```python
from build123d import *

# Parameters (mm, degrees)
BOSS_EXTRUDE1_DEPTH = 3.5
FILLET2_R           = 5
SHELL1_START        = 1
SHELL1_DEPTH        = 1.5
CUT_EXTRUDE1_START  = -3.5
SKETCH2_R           = 1
CUT_EXTRUDE1_DEPTH  = 3.5


# Read off the part's stored shape, not the designer's step: Shell1
with BuildPart() as part:
    # Sketch1 → Boss-Extrude1 (new body)
    with BuildSketch(Plane.XY):
        Polygon((0, 0), (-47, 0), (-47, 15), (-45, 15), (-45, 5.5), (0, 5.5), align=None)
    extrude(amount=BOSS_EXTRUDE1_DEPTH)

    # Fillet2
    fillet2_edges = [part.edges().sort_by_distance(p)[0] for p in [
        (-47, 0, 1.75),
        (-45, 5.5, 1.75),
    ]]
    fillet(fillet2_edges, radius=FILLET2_R)

    # Shell1 outline → Shell1 (cut)
    with BuildSketch(Plane.XY.offset(SHELL1_START)):
        with BuildLine():
            Line((0, 4.5), (-40, 4.5))
            ThreePointArc((-40, 4.5), (-44.242640687, 6.257359313), (-46, 10.5))
            Line((-46, 10.5), (-46, 5))
            ThreePointArc((-46, 5), (-44.828427125, 2.171572875), (-42, 1))
            Line((-42, 1), (0, 1))
            Line((0, 1), (0, 4.5))
        make_face()
    extrude(amount=SHELL1_DEPTH, mode=Mode.SUBTRACT)

    # Sketch2 → Cut-Extrude1 (cut)
    with BuildSketch(Plane.XY.offset(3.5).offset(CUT_EXTRUDE1_START)):
        with Locations(Location((-3, 2.75, 0), (0, 0, 180))):
            Circle(SKETCH2_R)
        with Locations(Location((-5.375, 2.75, 0), (0, 0, 180))):
            Circle(SKETCH2_R)
        with Locations(Location((-7.75, 2.75, 0), (0, 0, 180))):
            Circle(SKETCH2_R)
    extrude(amount=CUT_EXTRUDE1_DEPTH, mode=Mode.SUBTRACT)


solid = part.part
```
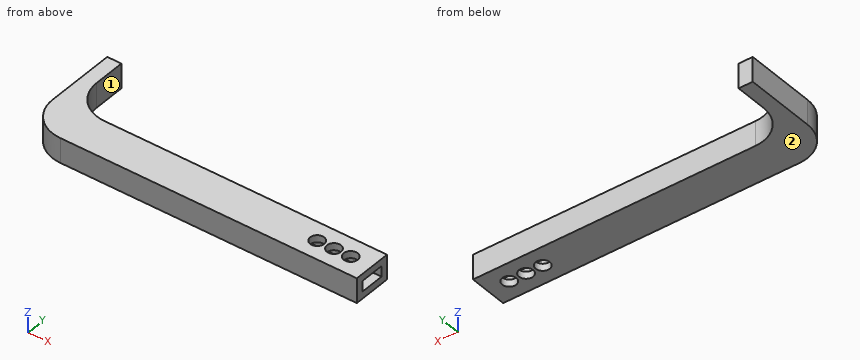
Work out the finished part from the listing and answer in its coordinate system (mm). Face numbers are marked on the shaded views. A direction names the side the tool comes from. Coordinates: 2 decimals unless noted, no trailing zeros. Write each loop counter-clockwise with the first axis right and the second up, starting at its lowest first coordinate (ties: lowest second). Pieces come first, ordered by that corner, then holes.
Q1. A cutting plane is placed at C-C, the plane z = 1.8. Give the vertices of the cut face in (x, y), then the cut area to 3 significant figures.
Q2. A cutting plane is placed at A-A, the plane x = -34.5. Give the vertices of the cut face in (y, z).
Q3. A cutting plane is placed at B-B, the plane y = 3.25. State how many separate pieces and enclosed holes the cut face has, then the cut area to 3 significant figures.
Q4. Which of the six approach directions +Z, -Z, +X, -X, +Y, -Y give full straight-line access (tool end or side, diameter ignored) to the marked faces 1 and 2?
Q5. Each of these flat-tipped pins is pushed along its axis until it touches: pin 1 Ø2.5 at (x, y) = (-3, 2.75) entering from -Z; pin 2 Ø1.8 at (x, z) = (-26.5, 2) entering from +Y; pin 3 Ø1.8 at (x, y) = (-5.375, 2.75) entering from +Z; pin 4 Ø1.2 at (y, z) = (7.5, 1.5) entering from +X. Where does it stop, or does it pass through?
Q6. Find the intervals of material crossed by line 1 (Y direction, x = -7.75, z = 3.15); line 2 (Y direction, x = -4, z = 1.95); line 3 (X direction, y = 2.75, z = 3.15) (3 decimals), in increasing order.
Q7. A cutting plane is placed at D-D, the plane x = -3. Give the vertices of the cut face in (y, z), then the cut area to 4 significant figures.
Findings below:
1. outline: (-47, 5) arc R5 ccw to (-42, 0) - (0, 0) - (0, 1) - (-42, 1) arc R4 cw to (-46, 5) - (-46, 10.5) arc R6 ccw to (-40, 4.5) - (0, 4.5) - (0, 5.5) - (-40, 5.5) arc R5 cw to (-45, 10.5) - (-45, 15) - (-47, 15) - close
1. area: 112 mm2
2. outline: (0, 0) - (5.5, 0) - (5.5, 3.5) - (0, 3.5) - close; hole (1, 1) - (4.5, 1) - (4.5, 2.5) - (1, 2.5) - close
3. separate pieces: 7
3. enclosed holes: 0
3. area: 84.6 mm2
4. face 1: +Z, -Z, +X, +Y
4. face 2: -Z, +X, -X, +Y, -Y
5. pin 1: stops at z = 0
5. pin 2: stops at y = 5.5
5. pin 3: passes through
5. pin 4: stops at x = -43.47
6. line 1: y = 0 to 1.75, 3.75 to 5.5
6. line 2: y = 0 to 1, 4.5 to 5.5
6. line 3: x = -46.465 to -8.75, -6.75 to -6.375, -4.375 to -4, -2 to 0
7. outline: (0, 0) - (1.75, 0) - (1.75, 1) - (1, 1) - (1, 2.5) - (1.75, 2.5) - (1.75, 3.5) - (0, 3.5) - close; (3.75, 0) - (5.5, 0) - (5.5, 3.5) - (3.75, 3.5) - (3.75, 2.5) - (4.5, 2.5) - (4.5, 1) - (3.75, 1) - close
7. area: 10.00 mm2
